The drawing under review shows one solid part. Ordinate dimensions are in mm from its lowest x, y, z. A direction names the side the tool comes from. Give positions to 0.01 mm unless a question says otherwise; leave off trailing zeros. Loops run counter-clockwise (first coordinate to the right, second up) from the corner with the lowest first, then second, coordinate; pieces in that order, holes last. Notation, with made-up numbers: (-26, 60.5) -> (-11, 60.5) arc R22 cw to (-11, 76.5) -> close; hole circle Ø8 at (35.25, 13.5). An arc over 180 degrees is marked (long way). Answer in a Markdown table with one row per item. Add a question column.
(1) For the marked faces 4, 5 and 6, list the 3-axis set-ups (+Z, -Z, +X, -X, +Y, -Y) from which the entire face can be reached by the end or side of a thin tool; tool diameter is ignored.
(2) Consider section A-A on y = 5. Write out the cut boundary in (x, z), then the cut area to 3 significant figures.
(3) Consider section B-B on x = 7.5. Write out the cut boundary in (y, z), then the cut area to 3 significant figures.
(4) For pin 1 (2 mm diameter, centred on y = 0.5, z = 6, fed in from -X); pin 2 (0.6 mm diameter, centred on x = 3.5, y = 1.5, fed in from +Z); pin 3 (0.9 mm diameter, centred on y = 3, z = 7, fed in from +X); pin 4 (6 mm diameter, centred on x = 5, y = 5, fed in from +Z), all flat-tipped, find the tip position at first contact; note any pin that passes through.
(5) Consider section D-D on y = 8.5. Write out the cut boundary in (x, z), then the cut area to 3 significant figures.
(6) Consider section C-C on z = 2.5. Write out the cut boundary in (x, y), then the cut area to 3 significant figures.
(7) For line 1 (Y direction, x = 5, z = 2); line 2 (X direction, y = 6.75, z = 5.5); line 3 (X direction, y = 5.5, z = 6.5), list the stretches that pass through material, from the lowest coordinate up.
(8) Draft analysis for pull direction X (two halves, no side actions). For the marked faces 1, 2 and 3, state which applies: +X half, -X half, draft (parallel to the pull), parting line (faces both ways), or undercut.
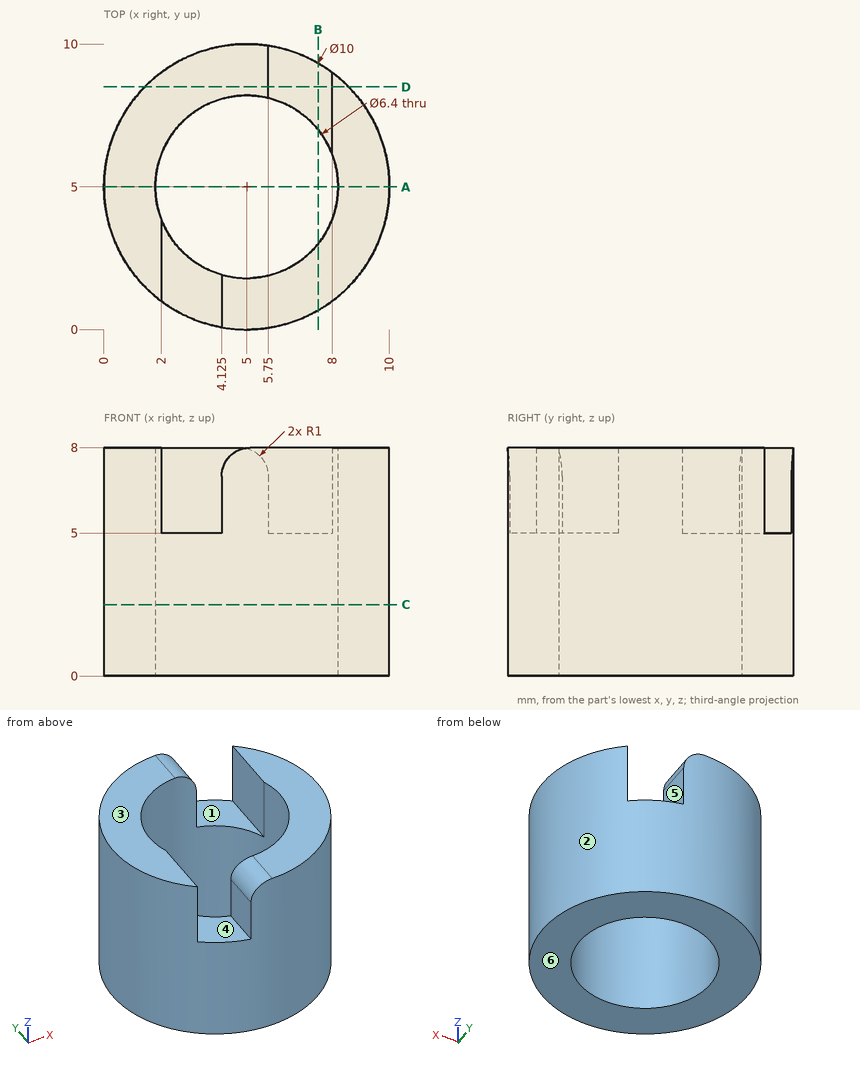
Values follow:
| question | item | result |
|---|---|---|
| 1 | face 4 | +Z, -Y |
| 1 | face 5 | +Z, +Y |
| 1 | face 6 | -Z, +X, -X, +Y, -Y |
| 2 | outline | (0, 0) -> (1.8, 0) -> (1.8, 8) -> (0, 8) -> close; (8.2, 0) -> (10, 0) -> (10, 8) -> (8.2, 8) -> close |
| 2 | area | 28.8 mm2 |
| 3 | outline | (0.67, 0) -> (3, 0) -> (3, 8) -> (0.67, 8) -> close; (7, 0) -> (9.33, 0) -> (9.33, 5) -> (7, 5) -> close |
| 3 | area | 30.3 mm2 |
| 4 | pin 1 | x = 1.43 |
| 4 | pin 2 | z = 5 |
| 4 | pin 3 | x = 9.75 |
| 4 | pin 4 | through |
| 5 | outline | (1.43, 0) -> (8.57, 0) -> (8.57, 8) -> (8, 8) -> (8, 5) -> (5.75, 5) -> (5.75, 7) arc R1 ccw to (4.75, 8) -> (1.43, 8) -> close |
| 5 | area | 50.2 mm2 |
| 6 | outline | circle Ø10 at (5, 5); hole circle Ø6.4 at (5, 5) |
| 6 | area | 46.4 mm2 |
| 7 | line 1 | 0 to 1.8, 8.2 to 10 |
| 7 | line 2 | 0.32 to 2.32, 8 to 9.68 |
| 7 | line 3 | 0.03 to 1.84, 8.16 to 9.97 |
| 8 | face 1 | undercut |
| 8 | face 2 | parting line |
| 8 | face 3 | draft |
